The model under review builds one solid part; all positions refer to its coordinate system, in mm. Round coordinates to 2 decimals unless told otherwise and drop trailing zeros. Order: outer loops, then holes, each group sorted by start corner. A loop starts at its lowest first (then second) coordinate and runs counter-clockwise, first axis right, second up. Notation, with made-up numbers: M -5.75,17 L 25.25,17 A15 cw 25.25,42 Z; hole C -38,82 d7. An arc over 180 degrees is marked long. Use a Markdown table: item, result. Add a question column.
1. To check wall thickness, follow probe 1 along Y at (x, z) = (0.1, 11.75); probe 2 along Z at (x, y) = (-2.45, -0.25). State the ranges of each line that lie inside material, in increasing order.
2. Consider section A-A on z = 12. State the section outline as (x, y) points.
3. Consider section B-B on x = -2.65. State the section outline as (y, z) points.
4. Insertion check: P1, Ø1, axis at x = -0.5, z = 13.5, coming from the -Y side; P2, Ø2, axis at x = -2.5, z = 5.5, coming from the +Y side. Each pin has a flat end and moves straight along its axis. Give the tip position at first contact, or say it passes through.
from build123d import *

# Parameters (mm, degrees)
F0_R     = 1.74
F1_DEPTH = 24.3
F2_SIZE2 = 0.655146
F2_SIZE  = 1.8
F3_R     = 1.05
F4_DEPTH = 4.23
F7_SIZE  = 0.2
F8_R     = 0.5


with BuildPart() as f1:
    # F0 (on Top) → F1 (new body)
    with BuildSketch(Plane.XY):
        Circle(F0_R)
    extrude(amount=F1_DEPTH)

    # F2
    f2_edges = [f1.edges().sort_by_distance(p)[0] for p in [
        (-1.74, 0, 24.3),
    ]]
    chamfer(f2_edges, length=F2_SIZE, length2=F2_SIZE2)

    # F3 (on Right) → F4 (join)
    with BuildSketch(Plane.YZ):
        with Locations((0, 1.831419)):
            Circle(F3_R)
    extrude(amount=-F4_DEPTH)

    # F5 (on Front) → F6 (revolve, cut)
    with BuildSketch(Plane.XZ):
        with BuildLine():
            Line((-3.08, 4.59), (-3.58, 4.59))
            Line((-3.58, 4.59), (-3.58, 2.89))
            ThreePointArc((-3.58, 2.89), (-3.33, 2.64), (-3.08, 2.89))
            Line((-3.08, 2.89), (-3.08, 4.59))
        make_face()
    revolve(axis=Axis((-4.23, 0, 1.831419), (1, 0, 0)), mode=Mode.SUBTRACT)

    # F7
    f7_edges = [f1.edges().sort_by_distance(p)[0] for p in [
        (-4.23, -1.05, 1.831419),
    ]]
    chamfer(f7_edges, length=F7_SIZE)

    # F8
    f8_edges = [f1.edges().sort_by_distance(p)[0] for p in [
        (-1.38748, -1.05, 1.831419),
    ]]
    fillet(f8_edges, radius=F8_R)


solid = f1.part
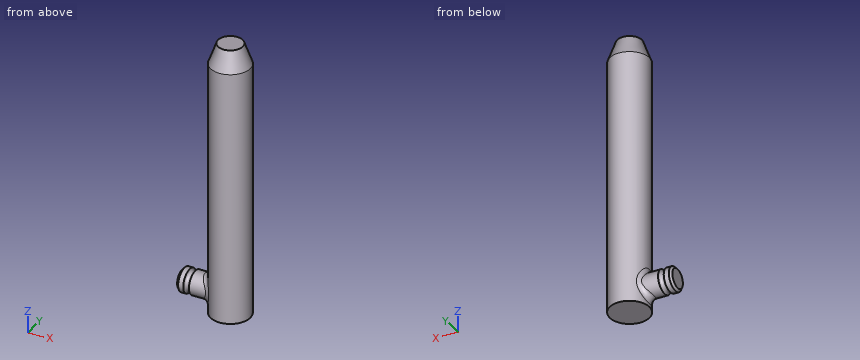
Answer block:
| question | item | result |
|---|---|---|
| 1 | probe 1 | -1.74 to 1.74 |
| 1 | probe 2 | 0.81 to 2.85 |
| 2 | outline | C 0,0 d3.48 |
| 3 | outline | C 0,1.83 d2.1 |
| 4 | P1 | y = -1.74 |
| 4 | P2 | y = 0.88 |
